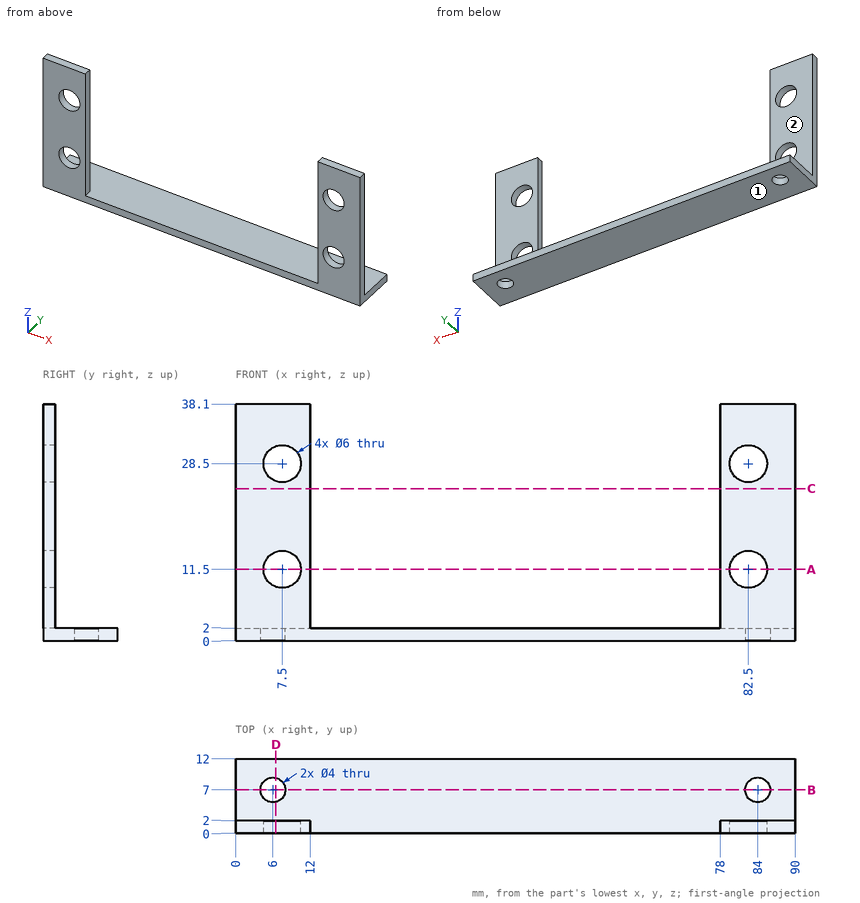
Design review of the part shown in the three views and the two pictorial views. Dimensions are in mm from the part's minimum x, y and z. A direction names the side the tool comes from. Give positions to 0.01 mm unless a question says otherwise; leave off trailing zeros. Order: outer loops, then holes, each group sorted by start corner. A loop starts at its lowest first (then second) coordinate and runs counter-clockwise, first axis right, second up. Notation, with made-up numbers: M -8,34 L 22,34 A15 ccw 22,52 Z; hole C -25,-29.5 d3. An arc over 180 degrees is marked long. Answer in a Markdown table with one row per item. Add a question column.
(1) Consider section C-C on z = 24.5. State the section outline as (x, y) points.
(2) For the marked faces 1 and 2, list the 3-axis set-ups (+Z, -Z, +X, -X, +Y, -Y) from which the entire face can be reached by the end or side of a thin tool; tool diameter is ignored.
(3) For pin 1 (5 mm diameter, centred on y = 5.5, z = 30.5, fed in from +X); pin 2 (6 mm diameter, centred on x = 42, y = 3, fed in from +Z); pin 3 (9.5 mm diameter, centred on x = 82.5, z = 11.5, fed in from +Y), all flat-tipped, find the tip position at first contact; note any pin that passes through.
(4) Wall thickness on probe 1 along X at (y, z) = (7, 1.1); probe 2 along X at (y, z) = (1.6, 11.5); probe 3 along Z at (x, y) = (63.5, 5): over which ranges is each line inside the solid? List them lowest first. Write a range as [from, to].
(5) Consider section D-D on x = 6.5. State the section outline as (y, z) points.
(6) Consider section B-B on y = 7. State the section outline as (x, z) points, and give its area (3 significant figures).
(7) Consider section A-A on z = 11.5. State the section outline as (x, y) points.
Evaluation:
| question | item | result |
|---|---|---|
| 1 | outline | M 0,0 L 12,0 L 12,2 L 0,2 Z; M 78,0 L 90,0 L 90,2 L 78,2 Z |
| 2 | face 1 | -Z, +X, -X, +Y, -Y |
| 2 | face 2 | +Z, +X, -X, +Y |
| 3 | pin 1 | passes through |
| 3 | pin 2 | stops at z = 2 |
| 3 | pin 3 | stops at y = 2 |
| 4 | probe 1 | x = [0, 4], [8, 82], [86, 90] |
| 4 | probe 2 | x = [0, 4.5], [10.5, 12], [78, 79.5], [85.5, 90] |
| 4 | probe 3 | z = [0, 2] |
| 5 | outline | M 0,0 L 5.06,0 L 5.06,2 L 2,2 L 2,8.67 L 0,8.67 Z; M 0,14.33 L 2,14.33 L 2,25.67 L 0,25.67 Z; M 0,31.33 L 2,31.33 L 2,38.1 L 0,38.1 Z; M 8.94,0 L 12,0 L 12,2 L 8.94,2 Z |
| 6 | outline | M 0,0 L 4,0 L 4,2 L 0,2 Z; M 8,0 L 82,0 L 82,2 L 8,2 Z; M 86,0 L 90,0 L 90,2 L 86,2 Z |
| 6 | area | 164 mm^2 |
| 7 | outline | M 0,0 L 4.5,0 L 4.5,2 L 0,2 Z; M 10.5,0 L 12,0 L 12,2 L 10.5,2 Z; M 78,0 L 79.5,0 L 79.5,2 L 78,2 Z; M 85.5,0 L 90,0 L 90,2 L 85.5,2 Z |
